```python
from build123d import *

# Parameters (mm, degrees)
BOSS_EXTRU_1_DEPTH = 8
CONG_1_R           = 3


with BuildPart() as part:
    # Esquisse1 → Boss.-Extru.1 (new body)
    with BuildSketch(Plane.XY):
        Polygon((-40.861442373, 48.763533187), (-15.861442373, 48.763533187), (-0.861442373, -3.236466813), (14.138557627, 48.763533187), (39.138557627, 48.763533187), (39.138557627, 40.763533187), (19.138557627, 40.763533187), (4.138557627, -11.236466813), (-5.861442373, -11.236466813), (-20.861442373, 40.763533187), (-40.861442373, 40.763533187), align=None)
    extrude(amount=BOSS_EXTRU_1_DEPTH)

    # Congé1
    cong_1_edges = [part.edges().sort_by_distance(p)[0] for p in [
        (-0.861442373, -3.236466813, 4),
    ]]
    fillet(cong_1_edges, radius=CONG_1_R)


solid = part.part
```
Read the model definition and answer for the solid it produces. Units are mm, in the model's axes. A direction names the side the tool comes from. Coordinates: 2 decimals unless noted, no trailing zeros. Write each loop counter-clockwise with the first axis right and the second up, starting at its lowest first coordinate (ties: lowest second). Pieces come first, ordered by that corner, then holes. Notation, with made-up numbers: (-9, 53) -> (43, 53) arc R25 ccw to (43, 69) -> close; hole circle Ø8 at (59.25, -38). An arc over 180 degrees is marked (long way). Return JSON: item names as keys, results as strings.
1. Each of these flat-tipped pins is pushed along its axis until it touches: P1, Ø2, axis at x = -5.5, y = 22, coming from the -Z side; P2, Ø2.5, axis at x = -35, z = 5, coming from the -Y side. Where does it stop, or does it pass through?
Found:
{"P1": "through", "P2": "y = 40.76"}
2. A cutting plane is placed at D-D (y = -6.5). Determine the outline of the cut face in (x, z), and give its area (3 significant figures).
Found:
{"outline": "(-7.23, 0) -> (5.5, 0) -> (5.5, 8) -> (-7.23, 8) -> close", "area": "102 mm2"}
3. A tool of negligible diameter and unlimited length cuts with its end or side. For faces 4 (the face through (-31, 40.764, 4)), 5 (the face through (29, 40.764, 4)), 6 (the face through (-9.9, 28.1, 3.9)), from which of +Z, -Z, +X, -X, +Y, -Y can it reach the whole face along a straight path? Write none if from no direction.
Found:
{"face 4": "+Z, -Z, -X, -Y", "face 5": "+Z, -Z, +X, -Y", "face 6": "+Z, -Z, +Y"}
4. A cutting plane is placed at C-C (x = -27). Determine the outline of the cut face in (y, z).
Found:
{"outline": "(40.76, 0) -> (48.76, 0) -> (48.76, 8) -> (40.76, 8) -> close"}
5. A cutting plane is placed at A-A (y = 31). Determine the outline of the cut face in (x, z).
Found:
{"outline": "(-18.05, 0) -> (-10.74, 0) -> (-10.74, 8) -> (-18.05, 8) -> close; (9.01, 0) -> (16.32, 0) -> (16.32, 8) -> (9.01, 8) -> close"}
6. Find the intervals of material crossed by line 1 along Y through (x, z) = (29, 0.5); line 2 along X through (y, z) = (44, 2.25); line 3 along X through (y, z) = (21.5, 4.25), in increasing order. Write a range as from..to.
Found:
{"line 1": "40.76..48.76", "line 2": "-40.86..-14.49, 12.76..39.14", "line 3": "-15.3..-8, 6.27..13.58"}
7. Determine the mould class of faces 1 (the face through (11.744, 15.128, 3.944)), 2 (the face through (-1, -11.236, 4)), 3 (the face through (7.995, 27.466, 3.944)) for opening direction X: pulls with the +X half, pulls with the -X half, needs draft (parallel to the pull), parting line crosses it, or undercut.
Found:
{"face 1": "pulls with the +X half", "face 2": "needs draft", "face 3": "undercut"}
8. A cutting plane is placed at B-B (z = 5.5). Determine the outline of the cut face in (x, y), and give its area (3 significant figures).
Found:
{"outline": "(-40.86, 40.76) -> (-20.86, 40.76) -> (-5.86, -11.24) -> (4.14, -11.24) -> (19.14, 40.76) -> (39.14, 40.76) -> (39.14, 48.76) -> (14.14, 48.76) -> (2.02, 6.76) arc R3 cw to (-3.74, 6.76) -> (-15.86, 48.76) -> (-40.86, 48.76) -> close", "area": "1,180 mm2"}
